Part model, mm, in its own coordinate system. A direction names the side the tool comes from. Give positions to 0.01 mm unless a question says otherwise; leave off trailing zeros. Write each loop counter-clockwise with the first axis right and the second up, starting at its lowest first coordinate (ties: lowest second). Pieces come first, ordered by that corner, then holes. Notation, with made-up numbers: (55, 57) - (59, 57) arc R25 ccw to (59, 91) - close; hole circle Ø7 at (-16.5, 49). An arc over 180 degrees is marked (long way). Answer as a JSON object with one key per item and string values. Group by question number.
```python
from build123d import *
from build123d.topology import SkipClean

# Parameters (mm, degrees)
SKETCH2_W                = 76
SKETCH2_H                = 12
BOSS_EXTRUDE1_DEPTH      = 55
BOSS_EXTRUDE2_DEPTH      = 7.5
BOSS_EXTRUDE3_DEPTH      = 10
BOSS_EXTRUDE3_DEPTH_BACK = 19
FILLET1_R                = 16
F_12_0MM_DOWEL_HOLE1_D   = 12
RIB1_START               = -3.75
RIB1_DEPTH               = 7.5
FILLET2_START            = 6
FILLET2_DEPTH            = 0.149958722
FILLET2_START_2          = 6.149958722
FILLET2_2_DEPTH          = 19.850041378
FILLET2_START_3          = -7.500000001
FILLET2_3_DEPTH          = 8.500000001


with BuildPart() as part:
    # Sketch2 → Boss-Extrude1 (new body)
    with BuildSketch(Plane(origin=(0, 0, 0), x_dir=(1, 0, 0), z_dir=(0, 1, 0))):
        Rectangle(SKETCH2_W, SKETCH2_H)
    extrude(amount=-BOSS_EXTRUDE1_DEPTH)

    # Sketch2<3> → Boss-Extrude2 (add)
    with BuildSketch(Plane(origin=(0, 0, 0), x_dir=(1, 0, 0), z_dir=(0, 1, 0))):
        with BuildLine():
            Line((18, -6), (-18, -6))
            Line((-18, -6), (-18, -84))
            ThreePointArc((-18, -84), (0, -66), (18, -84))
            Line((18, -84), (18, -6))
        make_face()
    extrude(amount=-BOSS_EXTRUDE2_DEPTH)

    # Sketch2<4> → Boss-Extrude3 (add, two sides: drawn at the far end of the back side and taken through both)
    with BuildSketch(Plane(origin=(0, 0, 0), x_dir=(1, 0, 0), z_dir=(0, 1, 0)).offset(-BOSS_EXTRUDE3_DEPTH_BACK)):
        with BuildLine():
            ThreePointArc((18, -84), (0, -66), (-18, -84))
            Line((-18, -84), (-6, -84))
            ThreePointArc((-6, -84), (0, -78), (6, -84))
            Line((6, -84), (18, -84))
        make_face()
        with BuildLine():
            Line((-6, -84), (-18, -84))
            ThreePointArc((-18, -84), (0, -102), (18, -84))
            Line((18, -84), (6, -84))
            ThreePointArc((6, -84), (0, -90), (-6, -84))
        make_face()
    extrude(amount=BOSS_EXTRUDE3_DEPTH + BOSS_EXTRUDE3_DEPTH_BACK)

    # Fillet1
    fillet1_edges = [part.edges().sort_by_distance(p)[0] for p in [
        (38, -55, 0),
        (-38, -55, 0),
        (-38, 0, 0),
        (38, 0, 0),
    ]]
    fillet(fillet1_edges, radius=FILLET1_R)

    # Ø12.0mm Dowel Hole1 (through all)
    with Locations(Plane.XY.offset(6)):
        with Locations((-22, -39), (22, -39)):
            Hole(F_12_0MM_DOWEL_HOLE1_D / 2)

    # Rib1: read off the stored shape, not the designer's step
    # Rib1 outline → Rib1 (add)
    with SkipClean():  # the faces are left unmerged after this step: merging them gives an invalid solid
        with BuildSketch(Plane.ZY.offset(RIB1_START)):
            Polygon((6, -55), (66.394958109, -18.763025135), (68, -17.8), (68, -7.5), (6, -7.5), align=None)
        extrude(amount=RIB1_DEPTH)

    # Fillet2: read off the stored shape, not the designer's step
    # Fillet2 outline → Fillet2 (add)
    with SkipClean():  # the faces are left unmerged after this step: merging them gives an invalid solid
        with BuildSketch(Plane.XY.offset(FILLET2_START)):
            with BuildLine():
                Line((-18, -7.5), (-18, 0))
                Line((-18, 0), (-22, 0))
                ThreePointArc((-22, 0), (-29.745966692, -2), (-35.555441712, -7.5))
                Line((-35.555441712, -7.5), (-18, -7.5))
            make_face()
            with BuildLine():
                Line((18, -7.5), (35.555441712, -7.5))
                ThreePointArc((35.555441712, -7.5), (29.745966692, -2), (22, 0))
                Line((22, 0), (18, 0))
                Line((18, 0), (18, -7.5))
            make_face()
        extrude(amount=FILLET2_DEPTH)

    # Fillet2 2 outline → Fillet2 2 (add)
    with SkipClean():  # the faces are left unmerged after this step: merging them gives an invalid solid
        with BuildSketch(Plane.XY.offset(FILLET2_START_2)):
            with BuildLine():
                Line((-18, -7.5), (-18, 0))
                Line((-18, 0), (-22, 0))
                ThreePointArc((-22, 0), (-29.745966693, -2), (-35.555441712, -7.500000001))
                Line((-35.555441712, -7.500000001), (-18, -7.5))
            make_face()
            with BuildLine():
                Line((18, -7.5), (35.555441712, -7.5))
                ThreePointArc((35.555441712, -7.5), (29.745966692, -2), (22, 0))
                Line((22, 0), (18, 0))
                Line((18, 0), (18, -7.5))
            make_face()
        extrude(amount=FILLET2_2_DEPTH)

    # Fillet2 3 outline → Fillet2 3 (cut)
    with SkipClean():  # the faces are left unmerged after this step: merging them gives an invalid solid
        with BuildSketch(Plane(origin=(0, 0, 0), x_dir=(1, 0, 0), z_dir=(0, 1, 0)).offset(FILLET2_START_3)):
            with BuildLine():
                Line((37, -5.972059597), (35.555441712, -6.149958822))
                ThreePointArc((35.555441712, -6.149958822), (23.018491969, -12.750305018), (18, -26))
                Line((18, -26), (37, -26.0000001))
                Line((37, -26.0000001), (37, -5.972059597))
            make_face()
            with BuildLine():
                Line((-35.555441712, -6.149958822), (-37, -5.972059597))
                Line((-37, -5.972059597), (-37, -26.0000001))
                Line((-37, -26.0000001), (-18, -26))
                ThreePointArc((-18, -26), (-23.018491969, -12.750305018), (-35.555441712, -6.149958822))
            make_face()
        extrude(amount=FILLET2_3_DEPTH, mode=Mode.SUBTRACT)


solid = part.part
```
1) Mould opens along X. For faces 4 (the cylindrical face through (-20.699, -44.857, -0.084)), 5 (the flat face through (-38, -27, 0)), 6 (the flat face through (38, -27, 0)) say: pulls with the +X half, pulls with the -X half, needs draft (parallel to the pull), parting line crosses it, or undercut.
2) Band-saw the part on A-A (z = 36). List the corners of the cut face in (x, y).
3) Band-saw the part on C-C (z = 85.5). List the corners of the cut face in (x, y), plus the area to 3 significant figures.
4) Probe line 1 (Z direction, x = 0, y = -8); line 2 (X direction, y = -14, z = 32); line 3 (Y direction, x = 11, z = 45.5). List the from-to ranges inside material, lowest first.
5) Which spindle directions (+Z, -Z, +X, -X, +Y, -Y) get a long thin tool onto all of the face, cutting with end or side? Do faces 1 (the flat face through (3.75, -26, 29)), 2 (the flat face through (-3.75, -26, 29)), 3 (the flat face through (-18, -4, 55)). Say none if no direction does.
6) Band-saw the part on B-B (y = -25). List the corners of the cut face in (x, z), plus the area to 3 significant figures.
7) Drop flat-ended pins along their axis: P1, Ø6, axis at y = -5, z = 65.5, coming from the -X side; P2, Ø6, axis at y = 0.5, z = 33.5, coming from the +X side; P3, Ø5, axis at x = 21.5, z = 30.5, coming from the -Y side; P4, Ø5, axis at y = -29.5, z = 22, coming from the -X side. Give the stop position or say it passes through.
8) Band-saw the part on D-D (z = 1.5). List the corners of the cut face in (x, y).
Verdict:
{
 "1": {"face 4": "undercut", "face 5": "pulls with the -X half", "face 6": "pulls with the +X half"},
 "2": {"outline": "(-18, -7.5) - (-3.75, -7.5) - (-3.75, -37) - (3.75, -37) - (3.75, -7.5) - (18, -7.5) - (18, 0) - (-18, 0) - close"},
 "3": {"outline": "(-17.94, -19) - (-5.81, -19) - (-5.81, 10) - (-17.94, 10) - close; (5.81, -19) - (17.94, -19) - (17.94, 10) - (5.81, 10) - close", "area": "703 mm2"},
 "4": {"line 1": "-6 to 78, 90 to 102", "line 2": "-3.75 to 3.75", "line 3": "-7.5 to 0"},
 "5": {"face 1": "+X, -Y", "face 2": "-X, -Y", "face 3": "+Z, -X, +Y, -Y"},
 "6": {"outline": "(-38, -6) - (38, -6) - (38, 6) - (3.75, 6) - (3.75, 56) - (-3.75, 56) - (-3.75, 6) - (-38, 6) - close", "area": "1,290 mm2"},
 "7": {"P1": "x = -18", "P2": "x = 18", "P3": "through", "P4": "x = -3.75"},
 "8": {"outline": "(-38, -39) arc R16 ccw to (-22, -55) - (22, -55) arc R16 ccw to (38, -39) - (38, -16) arc R16 ccw to (22, 0) - (-22, 0) arc R16 ccw to (-38, -16) - close; hole circle Ø12 at (-22, -39); hole circle Ø12 at (22, -39)"}
}
